The listing builds one solid part. Answer for the finished solid, in the listing's coordinates (mm). A direction names the side the tool comes from. Round coordinates to 2 decimals unless told otherwise and drop trailing zeros. Write each loop counter-clockwise with the first axis right and the second up, starting at its lowest first coordinate (ties: lowest second). Pieces come first, ordered by that corner, then holes. Notation, with made-up numbers: M 4,-26.75 L 14,-26.75 A8 cw 14,-16.75 Z; hole C -17,62.5 d3. An arc over 180 degrees is marked long. One line per item, written item: value. Start each with the question number.
(1) Section C-C (y = 8.5) is taken. Determine the outline of the cut face in (x, z).
(2) For a pull along X with two mould halves and no side action, classify faces 3 (the cylindrical face through (-5.158, 5.916, -3.955)), 4 (the cylindrical face through (1.617, 14.79, -0.67)), 5 (the flat face through (1, 40, 1)) as released by +X, released by -X, zero draft, split by the parting line, or undercut.
(3) Section A-A (x = 0) is taken. Determine the outline of the cut face in (y, z), plus the area to 3 significant figures.
(4) Given P1, Ø6, axis at y = 31, z = -26, coming from the -X side; P2, Ø4, axis at x = 18.5, y = 33, coming from the -Z side; P3, Ø12, axis at x = 3.5, y = 14.5, coming from the +Z side, each flat-ended and moving along its own axis, determine where each tip first touches the part or whether it passes through.
(5) For faces 1 (the flat face through (0, 30, 0)), 2 (the flat face through (1.4, 0, -1.4)), determine the directions among +Z, -Z, +X, -X, +Y, -Y from which every point of the face is accessible in a straight line to the end or side of a thin tool.
(6) Section D-D (y = 21) is taken. Determine the outline of the cut face in (x, z), plus the area to 3 significant figures.
(7) Consider probe 1 along Z at (x, y) = (0, 17); probe 2 along Z at (x, y) = (0, 11); probe 3 along Y at (x, z) = (1, 10.5). Determine where each line is inside the solid, lowest interval first.
(8) Section B-B (z = 0) is taken. Determine the outline of the cut face in (x, y).
```python
from build123d import *

# Parameters (mm, degrees)
F0_R     = 6.5
F0_R_2   = 1.75
F3_DEPTH = 20
F4_DEPTH = 30
F5_R     = 3


with BuildPart() as f2:
    # F1 (on Right) → F2 (revolve)
    with BuildSketch(Plane.YZ):
        Polygon((12, 20), (12, 0), (40, 0), (40, 38.768247), align=None)
    revolve(axis=Axis((0, 35.946441, 0), (0, 1, 0)))

    # F0 (on Front) → F3 (join)
    with BuildSketch(Plane.XZ):
        Circle(F0_R)
        Circle(F0_R_2, mode=Mode.SUBTRACT)
    extrude(amount=-F3_DEPTH)

    # F0 (on Front) → F4 (cut)
    with BuildSketch(Plane.XZ):
        Circle(F0_R_2)
    extrude(amount=-F4_DEPTH, mode=Mode.SUBTRACT)

    # F5
    f5_edges = [f2.edges().sort_by_distance(p)[0] for p in [
        (0, 12, -20),
    ]]
    fillet(f5_edges, radius=F5_R)


solid = f2.part
```
Recorded:
1. outline: C 0,0 d13; hole C 0,0 d3.5
2. face 3: split by the parting line
2. face 4: undercut
2. face 5: zero draft
3. outline: M 0,-6.5 L 12,-6.5 L 12,-18.4 A3 ccw 13.33,-20.89 L 40,-38.77 L 40,38.77 L 13.33,20.89 A3 ccw 12,18.4 L 12,6.5 L 0,6.5 L 0,1.75 L 30,1.75 L 30,-1.75 L 0,-1.75 Z
3. area: 1,700 mm2
4. P1: stops at x = -24.43
4. P2: stops at z = -30.6
4. P3: stops at z = 25.52
5. face 1: -Y
5. face 2: +Z, -Z, +X, -X, -Y
6. outline: C 0,0 d52.07; hole C 0,0 d3.5
6. area: 2,120 mm2
7. probe 1: z = -23.35 to -1.75, 1.75 to 23.35
7. probe 2: z = -6.5 to -1.75, 1.75 to 6.5
7. probe 3: y = 12 to 40
8. outline: M -38.77,40 L -20.89,13.33 A3 ccw -18.4,12 L -6.5,12 L -6.5,0 L -1.75,0 L -1.75,30 L 1.75,30 L 1.75,0 L 6.5,0 L 6.5,12 L 18.4,12 A3 ccw 20.89,13.33 L 38.77,40 Z
